CAD build for the part. Positions are in the model's coordinates, mm. A direction names the side the tool comes from. Give positions to 0.01 mm unless a question says otherwise; leave off trailing zeros. Loops run counter-clockwise (first coordinate to the right, second up) from the corner with the lowest first, then second, coordinate; pieces in that order, holes last.
```python
from build123d import *

# Parameters (mm, degrees)
F1_DEPTH = 3.048
F2_W     = 130.81
F2_H     = 178.816
F3_DEPTH = 25.4
F4_R     = 7.0104
F5_DEPTH = 25.4
F6_R     = 10.91242
F7_DEPTH = 5.08


with BuildPart() as f1:
    # F0 (on Top) → F1 (new body)
    with BuildSketch(Plane.XY):
        with BuildLine():
            ThreePointArc((-98.425, -100.838), (-90.985512, -118.798512), (-73.025, -126.238))
            Line((-73.025, -126.238), (73.025, -126.238))
            ThreePointArc((73.025, -126.238), (90.985512, -118.798512), (98.425, -100.838))
            Line((98.425, -100.838), (98.425, 100.838))
            ThreePointArc((98.425, 100.838), (90.985512, 118.798512), (73.025, 126.238))
            Line((73.025, 126.238), (-73.025, 126.238))
            ThreePointArc((-73.025, 126.238), (-90.985512, 118.798512), (-98.425, 100.838))
            Line((-98.425, 100.838), (-98.425, -100.838))
        make_face()
    extrude(amount=F1_DEPTH)

    # F2 (on face) → F3 (cut)
    with BuildSketch(Plane(origin=(0, 0, 0), x_dir=(1, 0, 0), z_dir=(0, 0, -1))):
        Rectangle(F2_W, F2_H)
    extrude(amount=-F3_DEPTH, mode=Mode.SUBTRACT)

    # F4 (on face) → F5 (cut)
    with BuildSketch(Plane(origin=(0, 0, 0), x_dir=(1, 0, 0), z_dir=(0, 0, -1))):
        with Locations((-81.915, 0)):
            Circle(F4_R)
        with Locations((81.915, 0)):
            Circle(F4_R)
    extrude(amount=-F5_DEPTH, mode=Mode.SUBTRACT)

    # F6 (on face) → F7 (join)
    with BuildSketch(Plane(origin=(0, 0, 0), x_dir=(1, 0, 0), z_dir=(0, 0, -1))):
        with Locations((78.195256, 104.103256)):
            Circle(F6_R)
        Polygon((72.54457, 105.392988), (75.680464, 109.325276), (80.710048, 109.325276), (83.845943, 105.392988), (82.726755, 100.489507), (78.195256, 98.307252), (73.663757, 100.489507), align=None, mode=Mode.SUBTRACT)
        with Locations((-78.195256, 104.103256)):
            Circle(F6_R)
        Polygon((-83.652061, 105.348736), (-80.623763, 109.146102), (-75.766749, 109.146102), (-72.738451, 105.348736), (-73.819238, 100.613498), (-78.195256, 98.506119), (-82.571274, 100.613498), align=None, mode=Mode.SUBTRACT)
        with Locations((-78.195256, -104.103256)):
            Circle(F6_R)
        Polygon((-83.845943, -102.813524), (-80.710048, -98.881237), (-75.680464, -98.881237), (-72.54457, -102.813524), (-73.663757, -107.717006), (-78.195256, -109.89926), (-82.726755, -107.717006), align=None, mode=Mode.SUBTRACT)
        with Locations((78.195256, -104.103256)):
            Circle(F6_R)
        Polygon((72.54457, -102.813524), (75.680464, -98.881237), (80.710048, -98.881237), (83.845943, -102.813524), (82.726755, -107.717006), (78.195256, -109.89926), (73.663757, -107.717006), align=None, mode=Mode.SUBTRACT)
    extrude(amount=F7_DEPTH)


solid = f1.part
```
1. Probe line 1 along X through (y, z) = (0, 0.8) (3 decimals); line 2 along X through (y, z) = (40, 2.75) (3 decimals); line 3 along Y through (x, z) = (-82, -1.25). List the from-to ranges inside material, lowest first.
Responses:
line 1: x = -98.425 to -88.925, -74.905 to -65.405, 65.405 to 74.905, 88.925 to 98.425
line 2: x = -98.425 to -65.405, 65.405 to 98.425
line 3: y = -114.33 to -107.42, -100.34 to -93.88, 93.88 to 100.5, 108.07 to 114.33
2. Saw through at D-D, the plane z = -2. Count the separate pieces of the cut face and the enclosed holes in it, and give its area (3 significant figures).
Responses:
separate pieces: 4
enclosed holes: 4
area: 1,130 mm2
3. Pull direction X, two halves, no side cores. Call faces 1 (the face through (90.79, -118.99, 1.5)), 2 (the face through (73, 106, -5.08)), 3 (the face through (-78, 98.881, -3)): released by +X, released by -X, zero draft, split by the parting line, or undercut.
Responses:
face 1: released by +X
face 2: zero draft
face 3: undercut
4. Drop flat-ended pins along their axis: pin 1 (3.5 mm diameter, centred on x = 81, y = -103.5, fed in from -Z); pin 2 (4 mm diameter, centred on x = 78.5, z = -3.5, fed in from +Y). Give the stop position or say it passes through.
Responses:
pin 1: stops at z = 0
pin 2: stops at y = 115.02
5. Saw through at A-A, the plane y = 0. List the corners of the cut face in (x, z) (3 decimals).
Responses:
outline: (-98.425, 0) - (-88.925, 0) - (-88.925, 3.048) - (-98.425, 3.048) - close; (-74.905, 0) - (-65.405, 0) - (-65.405, 3.048) - (-74.905, 3.048) - close; (65.405, 0) - (74.905, 0) - (74.905, 3.048) - (65.405, 3.048) - close; (88.925, 0) - (98.425, 0) - (98.425, 3.048) - (88.925, 3.048) - close
6. Saw through at B-B, the plane y = 44. List the corners of the cut face in (x, z) (3 decimals), and give its area (3 significant figures).
Responses:
outline: (-98.425, 0) - (-65.405, 0) - (-65.405, 3.048) - (-98.425, 3.048) - close; (65.405, 0) - (98.425, 0) - (98.425, 3.048) - (65.405, 3.048) - close
area: 201 mm2
7. Tool access for faces 4 (the face through (-81, 109, -5.08)), 5 (the face through (-78, 104, 0)): list every direction of +Z, -Z, +X, -X, +Y, -Y with a clear straight run to the whole face (end or side of a thin tool).
Responses:
face 4: -Z, +X, -X, +Y, -Y
face 5: -Z
8. Saw through at C-C, the plane x = -56. List the corners of the cut face in (y, z), and give its area (3 significant figures).
Responses:
outline: (-126.24, 0) - (-89.41, 0) - (-89.41, 3.05) - (-126.24, 3.05) - close; (89.41, 0) - (126.24, 0) - (126.24, 3.05) - (89.41, 3.05) - close
area: 225 mm2
